Source: three-view drawing plus pictorial views. Frame: mm from the lowest corner of the part. A direction names the side the tool comes from. Round coordinates to 2 decimals unless told otherwise and drop trailing zeros. Write each loop counter-clockwise with the first axis right and the second up, starting at its lowest first coordinate (ties: lowest second). Pieces come first, ordered by that corner, then holes. Notation, with made-up numbers: (-36, 11.5) -> (-2, 11.5) arc R17 ccw to (-2, 29.5) -> close; hole circle Ø1 at (57, 6). An arc over 180 degrees is marked (long way). Put each result on its own line as item: value.
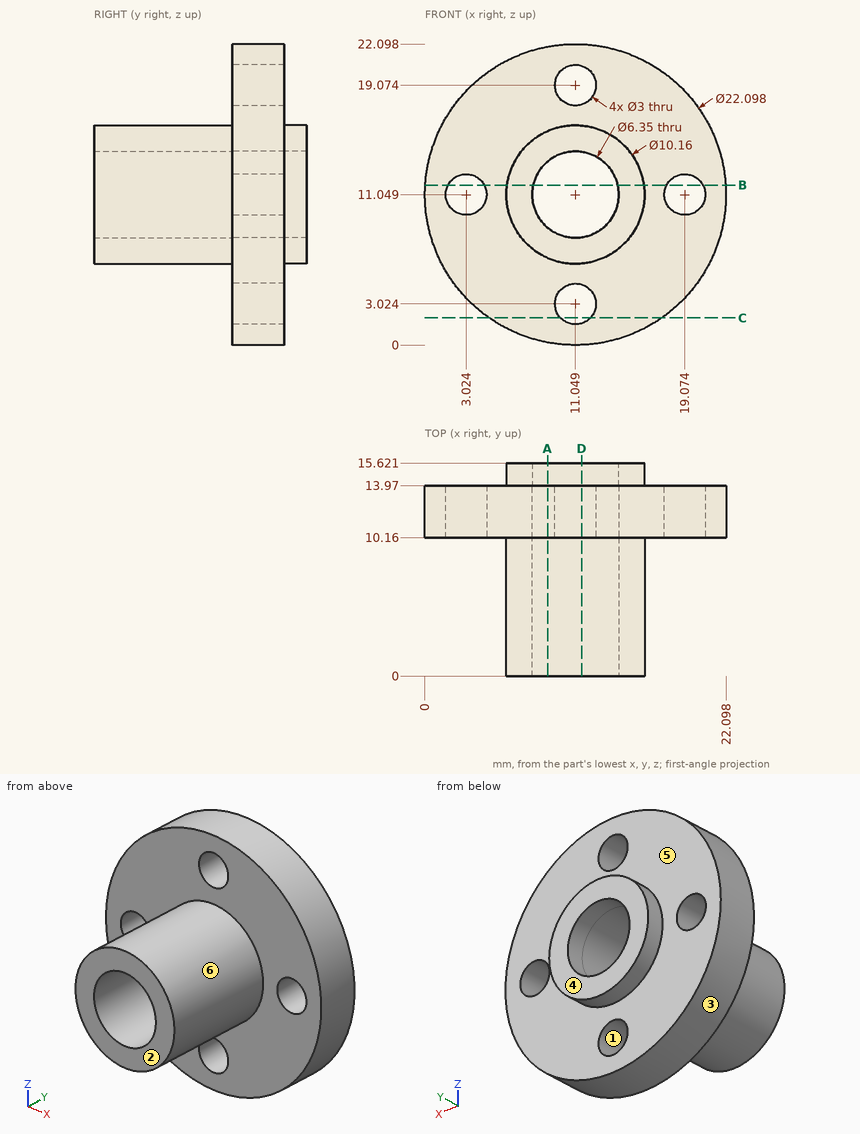
Q1. Cut plane B-B on z = 11.75. Output: boundary loops of the cut face in (x, y), and give its area (3 significant figures).
Ans:
outline: (0.02, 10.16) -> (1.7, 10.16) -> (1.7, 13.97) -> (0.02, 13.97) -> close; (4.35, 10.16) -> (6.02, 10.16) -> (6.02, 0) -> (7.95, 0) -> (7.95, 15.62) -> (6.02, 15.62) -> (6.02, 13.97) -> (4.35, 13.97) -> close; (14.15, 0) -> (16.08, 0) -> (16.08, 10.16) -> (17.75, 10.16) -> (17.75, 13.97) -> (16.08, 13.97) -> (16.08, 15.62) -> (14.15, 15.62) -> close; (20.4, 10.16) -> (22.08, 10.16) -> (22.08, 13.97) -> (20.4, 13.97) -> close
area: 85.9 mm^2
Q2. Cut plane C-C on z = 2. Output: boundary loops of the cut face in (x, y), and give its area (3 significant figures).
Ans:
outline: (4.71, 10.16) -> (9.95, 10.16) -> (9.95, 13.97) -> (4.71, 13.97) -> close; (12.15, 10.16) -> (17.39, 10.16) -> (17.39, 13.97) -> (12.15, 13.97) -> close
area: 40.0 mm^2
Q3. Pin query (flat end, axial travel): pin 1 (1.8 mm diameter, centred on x = 19.074, z = 11.049, fed in from +Y); pin 2 (1 mm diameter, centred on x = 16, y = 4.5, fed in from +Z); pin 3 (1 mm diameter, centred on x = 16.5, z = 17, fed in from -Y); pin 4 (3.5 mm diameter, centred on x = 11.049, z = 19.074, fed in from +Y). Return the tip coordinate at first contact, or that it passes through.
Ans:
pin 1: passes through
pin 2: stops at z = 13.5
pin 3: stops at y = 10.16
pin 4: stops at y = 13.97
Q4. Reachability of the marked faces 4, 5 and 6 from +Z, -Z, +X, -X, +Y, -Y: full face, straight path, thin tool, end or side. Return the list, or none.
Ans:
face 4: +Z, -Z, +X, -X, +Y
face 5: +Y
face 6: -Y
Q5. Material intervals for line 1 (Z direction, x = 11.25, y = 12); line 2 (X direction, y = 1.5, z = 11); line 3 (Y direction, x = 1, z = 7.5), sorted ascending. Write a range as [from, to].
Ans:
line 1: z = [0, 1.54], [4.51, 7.88], [14.22, 17.59], [20.56, 22.1]
line 2: x = [5.97, 7.87], [14.22, 16.13]
line 3: y = [10.16, 13.97]
Q6. Draft query along X for the marked faces 1, 2 and 3. Return one class per face: +X half, -X half, draft (parallel to the pull), parting line (faces both ways), or undercut.
Ans:
face 1: undercut
face 2: draft
face 3: parting line
Q7. Cut plane D-D on x = 11.5. Output: boundary loops of the cut face in (y, z), and give its area (3 significant figures).
Ans:
outline: (0, 5.99) -> (10.16, 5.99) -> (10.16, 4.45) -> (13.97, 4.45) -> (13.97, 5.99) -> (15.62, 5.99) -> (15.62, 7.91) -> (0, 7.91) -> close; (0, 14.19) -> (15.62, 14.19) -> (15.62, 16.11) -> (13.97, 16.11) -> (13.97, 17.64) -> (10.16, 17.64) -> (10.16, 16.11) -> (0, 16.11) -> close; (10.16, 0.01) -> (13.97, 0.01) -> (13.97, 1.59) -> (10.16, 1.59) -> close; (10.16, 20.5) -> (13.97, 20.5) -> (13.97, 22.09) -> (10.16, 22.09) -> close
area: 83.7 mm^2
Q8. Cut plane A-A on x = 9. Output: boundary loops of the cut face in (y, z), and give its area (3 significant figures).
Ans:
outline: (0, 6.4) -> (10.16, 6.4) -> (10.16, 0.19) -> (13.97, 0.19) -> (13.97, 6.4) -> (15.62, 6.4) -> (15.62, 8.62) -> (0, 8.62) -> close; (0, 13.47) -> (15.62, 13.47) -> (15.62, 15.7) -> (13.97, 15.7) -> (13.97, 21.91) -> (10.16, 21.91) -> (10.16, 15.7) -> (0, 15.7) -> close
area: 117 mm^2
